```python
from build123d import *

# Parameters (mm, degrees)
BOSS_EXTRUDE1_DEPTH = 2
SKETCH2_R           = 35
CUT_EXTRUDE1_DEPTH  = 85.718414298
SKETCH4_R           = 1.5
CUT_EXTRUDE3_DEPTH  = 2
SKETCH5_W           = 23
SKETCH5_H           = 3
CUT_EXTRUDE4_DEPTH  = 85.718414298


with BuildPart() as part:
    # Sketch1 → Boss-Extrude1 (new body)
    with BuildSketch(Plane.XY):
        with BuildLine():
            Line((21.520746486, 52.119258472), (15.256667967, 42.372162038))
            Line((15.256667967, 42.372162038), (32.20522538, 31.479985569))
            Line((32.20522538, 31.479985569), (38.4693039, 41.227082003))
            ThreePointArc((38.4693039, 41.227082003), (40.698070229, 42.590620718), (43.150594208, 41.689641633))
            ThreePointArc((43.150594208, 41.689641633), (45.344974461, 39.291644037), (47.406271028, 36.778328771))
            ThreePointArc((47.406271028, 36.778328771), (47.949048893, 34.222545257), (46.282202516, 32.210516346))
            Line((46.282202516, 32.210516346), (35.742846148, 27.397353567))
            Line((35.742846148, 27.397353567), (44.112124759, 9.071189697))
            Line((44.112124759, 9.071189697), (54.651481127, 13.884352476))
            ThreePointArc((54.651481127, 13.884352476), (57.263623361, 13.826472187), (58.839711753, 11.742585779))
            ThreePointArc((58.839711753, 11.742585779), (59.389286513, 8.538890296), (59.764558712, 5.310133889))
            ThreePointArc((59.764558712, 5.310133889), (58.83941162, 2.86662411), (56.349386262, 2.075162869))
            Line((56.349386262, 2.075162869), (44.880923224, 3.724078919))
            Line((44.880923224, 3.724078919), (42.013736207, -16.217644809))
            Line((42.013736207, -16.217644809), (53.482199245, -17.86656086))
            ThreePointArc((53.482199245, -17.86656086), (55.648380681, -19.32748357), (55.847636558, -21.93265809))
            ThreePointArc((55.847636558, -21.93265809), (54.577919721, -24.92490078), (53.148021281, -27.843990983))
            ThreePointArc((53.148021281, -27.843990983), (51.048676897, -29.399429937), (48.526038015, -28.719040157))
            Line((48.526038015, -28.719040157), (39.76962429, -21.131564473))
            Line((39.76962429, -21.131564473), (26.576283265, -36.357491677))
            Line((26.576283265, -36.357491677), (35.33269699, -43.944967362))
            ThreePointArc((35.33269699, -43.944967362), (36.365170327, -46.345099856), (35.124331356, -48.644437984))
            ThreePointArc((35.124331356, -48.644437984), (32.438449047, -50.47521197), (29.657362619, -52.157845455))
            ThreePointArc((29.657362619, -52.157845455), (27.050347952, -52.331372705), (25.296015568, -50.395150852))
            Line((25.296015568, -50.395150852), (22.031750643, -39.278085453))
            Line((22.031750643, -39.278085453), (2.701048165, -44.954091828))
            Line((2.701048165, -44.954091828), (5.96531309, -56.071157227))
            ThreePointArc((5.96531309, -56.071157227), (5.536275339, -58.648474396), (3.249299125, -59.911952524))
            ThreePointArc((3.249299125, -59.911952524), (0, -60), (-3.249299125, -59.911952524))
            ThreePointArc((-3.249299125, -59.911952524), (-5.536275339, -58.648474396), (-5.96531309, -56.071157227))
            Line((-5.96531309, -56.071157227), (-2.701048165, -44.954091828))
            Line((-2.701048165, -44.954091828), (-22.031750643, -39.278085453))
            Line((-22.031750643, -39.278085453), (-25.296015568, -50.395150852))
            ThreePointArc((-25.296015568, -50.395150852), (-27.050347952, -52.331372705), (-29.657362619, -52.157845455))
            ThreePointArc((-29.657362619, -52.157845455), (-32.438449047, -50.47521197), (-35.124331356, -48.644437984))
            ThreePointArc((-35.124331356, -48.644437984), (-36.365170327, -46.345099856), (-35.33269699, -43.944967362))
            Line((-35.33269699, -43.944967362), (-26.576283265, -36.357491677))
            Line((-26.576283265, -36.357491677), (-39.76962429, -21.131564473))
            Line((-39.76962429, -21.131564473), (-48.526038015, -28.719040157))
            ThreePointArc((-48.526038015, -28.719040157), (-51.048676897, -29.399429937), (-53.148021281, -27.843990983))
            ThreePointArc((-53.148021281, -27.843990983), (-54.577919721, -24.92490078), (-55.847636558, -21.93265809))
            ThreePointArc((-55.847636558, -21.93265809), (-55.648380681, -19.32748357), (-53.482199245, -17.86656086))
            Line((-53.482199245, -17.86656086), (-42.013736207, -16.217644809))
            Line((-42.013736207, -16.217644809), (-44.880923224, 3.724078919))
            Line((-44.880923224, 3.724078919), (-56.349386262, 2.075162869))
            ThreePointArc((-56.349386262, 2.075162869), (-58.83941162, 2.86662411), (-59.764558712, 5.310133889))
            ThreePointArc((-59.764558712, 5.310133889), (-59.389286513, 8.538890296), (-58.839711753, 11.742585779))
            ThreePointArc((-58.839711753, 11.742585779), (-57.263623361, 13.826472187), (-54.651481127, 13.884352476))
            Line((-54.651481127, 13.884352476), (-44.112124759, 9.071189697))
            Line((-44.112124759, 9.071189697), (-35.742846148, 27.397353567))
            Line((-35.742846148, 27.397353567), (-46.282202516, 32.210516346))
            ThreePointArc((-46.282202516, 32.210516346), (-47.949048893, 34.222545257), (-47.406271028, 36.778328771))
            ThreePointArc((-47.406271028, 36.778328771), (-45.344974461, 39.291644037), (-43.150594208, 41.689641633))
            ThreePointArc((-43.150594208, 41.689641633), (-40.698070229, 42.590620718), (-38.4693039, 41.227082003))
            Line((-38.4693039, 41.227082003), (-32.20522538, 31.479985569))
            Line((-32.20522538, 31.479985569), (-15.256667967, 42.372162038))
            Line((-15.256667967, 42.372162038), (-21.520746486, 52.119258472))
            ThreePointArc((-21.520746486, 52.119258472), (-21.835201934, 54.713050089), (-19.99682725, 56.569664131))
            ThreePointArc((-19.99682725, 56.569664131), (-16.90395341, 57.569578417), (-13.76146789, 58.400530832))
            ThreePointArc((-13.76146789, 58.400530832), (-11.211167359, 57.832548102), (-10.073394495, 55.480504291))
            Line((-10.073394495, 55.480504291), (-10.073394495, 43.894108449))
            Line((-10.073394495, 43.894108449), (10.073394495, 43.894108449))
            Line((10.073394495, 43.894108449), (10.073394495, 55.480504291))
            ThreePointArc((10.073394495, 55.480504291), (11.211167359, 57.832548102), (13.76146789, 58.400530832))
            ThreePointArc((13.76146789, 58.400530832), (16.90395341, 57.569578417), (19.99682725, 56.569664131))
            ThreePointArc((19.99682725, 56.569664131), (21.835201934, 54.713050089), (21.520746486, 52.119258472))
        make_face()
    extrude(amount=BOSS_EXTRUDE1_DEPTH)

    # Sketch2 → Cut-Extrude1 (cut, through all)
    with BuildSketch(Plane.XY.offset(2)):
        Circle(SKETCH2_R)
    extrude(amount=-CUT_EXTRUDE1_DEPTH, mode=Mode.SUBTRACT)

    # Sketch4 → Cut-Extrude3 (cut)
    with BuildSketch(Plane.XY.offset(2)):
        with Locations((-14.086627842, 47.974648681)):
            Circle(SKETCH4_R)
        with Locations((14.086627842, 47.974648681)):
            Circle(SKETCH4_R)
        with Locations((37.787478718, 32.743036697)):
            Circle(SKETCH4_R)
        with Locations((49.491072094, 7.115741914)):
            Circle(SKETCH4_R)
        with Locations((45.481599768, -20.77075065)):
            Circle(SKETCH4_R)
        with Locations((27.032040873, -42.062676642)):
            Circle(SKETCH4_R)
        with Locations((0, -50)):
            Circle(SKETCH4_R)
        with Locations((-27.032040873, -42.062676642)):
            Circle(SKETCH4_R)
        with Locations((-45.481599768, -20.77075065)):
            Circle(SKETCH4_R)
        with Locations((-49.491072094, 7.115741914)):
            Circle(SKETCH4_R)
        with Locations((-37.787478718, 32.743036697)):
            Circle(SKETCH4_R)
    extrude(amount=-CUT_EXTRUDE3_DEPTH, mode=Mode.SUBTRACT)

    # Sketch5 → Cut-Extrude4 (cut, through all)
    with BuildSketch(Plane.XY.offset(2)):
        Polygon((20.331149741, 52.906940473), (18.709227289, 50.383179874), (38.058058544, 37.948441073), (39.679980996, 40.472201671), align=None)
        with Locations((0, 54)):
            Rectangle(SKETCH5_W, SKETCH5_H)
        Polygon((45.707303093, 33.516301168), (42.978407107, 32.270056129), (52.532952406, 11.348520236), (55.261848392, 12.594765275), align=None)
        Polygon((56.571710665, 3.484473057), (53.602246339, 3.911417572), (50.329005059, -18.854475591), (53.298469384, -19.281420106), align=None)
        Polygon((49.474999817, -27.653650629), (47.207751094, -25.689068427), (32.145954213, -43.071308637), (34.413202936, -45.035890839), align=None)
        Polygon((26.670326101, -50.011935632), (25.825128431, -47.133456711), (3.756790038, -53.613305518), (4.601987708, -56.491784439), align=None)
        Polygon((-4.601987708, -56.491784439), (-3.756790038, -53.613305518), (-25.825128431, -47.133456711), (-26.670326101, -50.011935632), align=None)
        Polygon((-34.413202936, -45.035890839), (-32.145954213, -43.071308637), (-47.207751094, -25.689068427), (-49.474999817, -27.653650629), align=None)
        Polygon((-53.298469384, -19.281420106), (-50.329005059, -18.854475591), (-53.602246339, 3.911417572), (-56.571710665, 3.484473057), align=None)
        Polygon((-55.261848392, 12.594765275), (-52.532952406, 11.348520236), (-42.978407107, 32.270056129), (-45.707303093, 33.516301168), align=None)
        Polygon((-39.679980996, 40.472201671), (-38.058058544, 37.948441073), (-18.709227289, 50.383179874), (-20.331149741, 52.906940473), align=None)
    extrude(amount=-CUT_EXTRUDE4_DEPTH, mode=Mode.SUBTRACT)


solid = part.part
```
Can you work these out from the model? Positions are in its coordinate system, mm. A direction names the side the tool comes from. Give positions to 0.01 mm unless a question says otherwise; leave off trailing zeros. Order: outer loops, then holes, each group sorted by start corner. A loop starts at its lowest first (then second) coordinate and runs counter-clockwise, first axis right, second up. Notation, with made-up numbers: M 69,55.5 L 97,55.5 A19 ccw 97,73.5 Z; hole C -21,-5.5 d11. An arc over 180 degrees is marked long. Write item = value, one per line. Start each with the question number.
Q1. I need wall thicknesses on probe 1 along Y at (x, z) = (0, 1.05); probe 2 along Y at (x, z) = (-29.5, 1.1); probe 3 along Y at (x, z) = (-19.5, 1.55). Which ranges of each line are inside material? Lowest first, please. Write a range as [from, to].
Q2. Suppose I cut it at C-C (x = -17). Write out the boundary of the cut face in (y, z).
Q3. Suppose I cut it at A-A (x = 0). Write out the boundary of the cut face in (y, z).
Q4. For faces 5 (the flat face through (43.07, -23.99, 0.99)), 6 (the flat face through (-33.08, -28.85, 0.99)), 7 (the flat face through (34.5, 35.05, 0.99)), which set-ups out of +Z, -Z, +X, -X, +Y, -Y let a thin tool reach every point of the face, with its end or its side?
Q5. We'd pull the mould along X, two halves only. Please class faces 1 (the flat face through (-39.6, 29.16, 0.99)), 2 (the flat face through (39.87, 18.36, 0.99)), 3 (the cylindrical face through (44, -21, 1)), 4 (the cylindrical face through (5.55, -58.63, 0.99)): pulls with the +X half, pulls with the -X half, needs draft (parallel to the pull), parting line crosses it, or undercut.
Q6. Will these pins go through, and if not, where does the flat tip stop? pin 1 Ø1 at (y, z) = (-4, 1.5) entering from -X; pin 2 Ø1.8 at (x, y) = (45.48, -20.77) entering from -Z; pin 3 Ø1 at (y, z) = (-10.5, 0.5) entering from -X; pin 4 Ø1 at (y, z) = (47.5, 1) entering from -X.
Q7. Suppose I cut it at B-B (y = 0). Write out the boundary of the cut face in (x, z).
Q8. Suppose I cut it at D-D (z = 1.25). Count the separate pieces of the cut face and the enclosed holes in it, plus the area to 3 significant figures.
Check result:
q1.probe_1 = [-60, -51.5], [-48.5, -35], [35, 43.89]
q1.probe_2 = [-52.24, -38.89], [-32.98, -18.83], [18.83, 33.22]
q1.probe_3 = [-40.02, -29.06], [29.06, 39.65], [48.97, 49.87], [51.61, 56.74]
q2.outline = M -40.76,0 L -30.59,0 L -30.59,2 L -40.76,2 Z; M 30.59,0 L 41.25,0 L 41.25,2 L 30.59,2 Z; M 45.08,0 L 57.54,0 L 57.54,2 L 45.08,2 Z
q3.outline = M -60,0 L -51.5,0 L -51.5,2 L -60,2 Z; M -48.5,0 L -35,0 L -35,2 L -48.5,2 Z; M 35,0 L 43.89,0 L 43.89,2 L 35,2 Z
q4.face_5 = +Z, -Z, -Y
q4.face_6 = +Z, -Z
q4.face_7 = +Z, -Z, +Y
q5.face_1 = pulls with the -X half
q5.face_2 = undercut
q5.face_3 = undercut
q5.face_4 = pulls with the +X half
q6.pin_1 = -43.84
q6.pin_2 = through
q6.pin_3 = -42.91
q6.pin_4 = -18.87
q7.outline = M -44.35,0 L -35,0 L -35,2 L -44.35,2 Z; M 35,0 L 44.35,0 L 44.35,2 L 35,2 Z
q8.separate_pieces = 1
q8.enclosed_holes = 12
q8.area = 3,710 mm2
